Source: CAD feature listing. Evaluate the final solid. Frame: model axes, mm. Face numbers are marked on the shaded views. A direction names the side the tool comes from. Give positions to 0.01 mm unless a question says otherwise; leave off trailing zeros. Order: outer loops, then holes, each group sorted by start corner. A loop starts at its lowest first (then second) coordinate and runs counter-clockwise, first axis right, second up. Notation, with made-up numbers: M 86,-3.75 L 134,-3.75 A21 ccw 134,18.25 Z; hole C -17.5,38.5 d6. An arc over 180 degrees is marked long. Return JSON: item names as keys, results as strings.
from build123d import *

# Parameters (mm, degrees)
EXTRUDE_1_DEPTH             = 60
CUT_EXTRUDE_1_DEPTH         = 4
SKETCH_3_W                  = 5
SKETCH_3_H                  = 5
CUT_EXTRUDE_2_DEPTH         = 4
FILLET_1_R                  = 2
FILLET_2_R                  = 1
HOLE_WIZARD_M31_D           = 3.4
HOLE_WIZARD_M31_CBORE_D     = 6.5
HOLE_WIZARD_M31_CBORE_DEPTH = 3
SKETCH_9_W                  = 16.027024291
SKETCH_9_H                  = 8.780763308
CUT_EXTRUDE_4_DEPTH         = 6
SKETCH_10_R                 = 1.700955844
CUT_EXTRUDE_5_DEPTH         = 68.823299831


with BuildPart() as part:
    # Эскиз1 → Бобышка-Вытянуть1 (new body)
    with BuildSketch(Plane.XY):
        Polygon((-20, 5), (-15.381197846, -3), (-15.381197846, -4), (-30, -4), (-30, -6), (30, -6), (30, -4), (15.381197846, -4), (15.381197846, -3), (20, 5), (20, 6), (-20, 6), align=None)
    extrude(amount=EXTRUDE_1_DEPTH)

    # Эскиз2 → Вырез-Вытянуть1 (cut)
    with BuildSketch(Plane(origin=(0, 6, 0), x_dir=(1, 0, 0), z_dir=(0, 1, 0))):
        Polygon((15, 0), (-15, 0), (-15, -5), (-10.336923418, -15), (-10.336923418, -45), (-15, -55), (-15, -60), (15, -60), (15, -55), (10.336923418, -45), (10.336923418, -15), (15, -5), align=None)
    extrude(amount=-CUT_EXTRUDE_1_DEPTH, mode=Mode.SUBTRACT)

    # Эскиз3 → Вырез-Вытянуть2 (cut)
    with BuildSketch(Plane(origin=(0, 6, 0), x_dir=(1, 0, 0), z_dir=(0, 1, 0))):
        with Locations((-12.836923418, -30)):
            Rectangle(SKETCH_3_W, SKETCH_3_H)
        with Locations((12.836923418, -30)):
            Rectangle(SKETCH_3_W, SKETCH_3_H)
    extrude(amount=-CUT_EXTRUDE_2_DEPTH, mode=Mode.SUBTRACT)

    # Скругление1
    fillet_1_edges = [part.edges().sort_by_distance(p)[0] for p in [
        (20, 5.5, 0),
        (-20, 5.5, 0),
        (20, 5.5, 60),
        (-20, 5.5, 60),
        (-15, 4, 5),
        (-15, 4, 0),
        (15, 4, 0),
        (15, 4, 5),
        (10.336923418, 4, 15),
        (10.336923418, 4, 45),
        (15, 4, 55),
        (15, 4, 60),
        (-15, 4, 60),
        (-15, 4, 55),
    ]]
    fillet(fillet_1_edges, radius=FILLET_1_R)

    # Скругление2
    fillet_2_edges = [part.edges().sort_by_distance(p)[0] for p in [
        (-15.336923418, 4, 32.5),
        (-15.336923418, 4, 27.5),
        (10.336923418, 4, 27.5),
        (15.336923418, 4, 27.5),
        (15.336923418, 4, 32.5),
        (10.336923418, 4, 32.5),
    ]]
    fillet(fillet_2_edges, radius=FILLET_2_R)

    # Цековка для винта с внутренним шестигранником M31 (through all)
    with Locations(Plane(origin=(0, 2, 0), x_dir=(1, 0, 0), z_dir=(0, 1, 0))):
        with Locations((0, -24), (6, -30), (0, -36), (-6, -30)):
            CounterBoreHole(HOLE_WIZARD_M31_D / 2, HOLE_WIZARD_M31_CBORE_D / 2, HOLE_WIZARD_M31_CBORE_DEPTH)

    # Эскиз9 → Вырез-Вытянуть4 (cut)
    with BuildSketch(Plane(origin=(0, 2, 0), x_dir=(1, 0, 0), z_dir=(0, 1, 0))):
        with Locations((1.449252196, -53.358535403)):
            Rectangle(SKETCH_9_W, SKETCH_9_H)
    extrude(amount=-CUT_EXTRUDE_4_DEPTH, mode=Mode.SUBTRACT)

    # Эскиз10 → Вырез-Вытянуть5 (cut, through all)
    with BuildSketch(Plane(origin=(0, -4, 0), x_dir=(1, 0, 0), z_dir=(0, 1, 0))):
        with Locations(Location((-4.749733233, -52.305802454, 0), (0, 0, 180))):
            Circle(SKETCH_10_R)
    extrude(amount=-CUT_EXTRUDE_5_DEPTH, mode=Mode.SUBTRACT)


solid = part.part
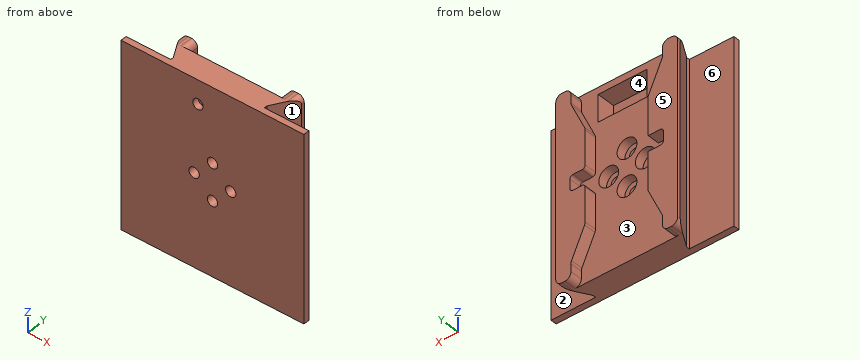
1. Draft query along X for the marked faces 1, 2, 3 and 4. Return one class per face: pulls with the +X half, pulls with the -X half, needs draft (parallel to the pull), parting line crosses it, or undercut.
Evaluation:
{"face 1": "pulls with the +X half", "face 2": "needs draft", "face 3": "undercut", "face 4": "undercut"}
2. Section query D-D (z = 13). Return loops of the section in (x, y).
Evaluation:
{"outline": "M -30,-6 L 30,-6 L 30,-4 L 15.38,-4 L 15.38,-3 L 20,5 L 20,6 L 11.27,6 L 11.27,2 L -11.27,2 L -11.27,6 L -20,6 L -20,5 L -15.38,-3 L -15.38,-4 L -30,-4 Z"}
3. Section query C-C (z = 37). Return loops of the section in (x, y), then the cut area to 3 significant figures.
Evaluation:
{"outline": "M -30,-6 L -1.37,-6 L -1.37,-1 L -3.09,-1 L -3.09,2 L -10.34,2 L -10.34,6 L -20,6 L -20,5 L -15.38,-3 L -15.38,-4 L -30,-4 Z; M 1.37,-6 L 30,-6 L 30,-4 L 15.38,-4 L 15.38,-3 L 20,5 L 20,6 L 10.34,6 L 10.34,2 L 3.09,2 L 3.09,-1 L 1.37,-1 Z", "area": "359 mm^2"}
4. Section query B-B (z = 30). State how many separate pieces and enclosed holes the cut face has, then the cut area to 3 significant figures.
Evaluation:
{"separate pieces": "3", "enclosed holes": "0", "area": "278 mm^2"}
5. Ray query, probe 1 along X at (y, z) = (-3.65, 30); probe 2 along Z at (x, y) = (-6, -0.2); probe 3 along Z at (x, y) = (6, -4.2). Return the intervals inside material, ascending.
Evaluation:
{"probe 1": "x = -15.38 to -7.7, -4.3 to 4.3, 7.7 to 15.38", "probe 2": "z = 0 to 26.75, 33.25 to 48.97, 57.75 to 60", "probe 3": "z = 0 to 28.3, 31.7 to 60"}
6. First-contact query: pin 1 (5 mm diameter, centred on y = 4.5, z = 46, fed in from -X); pin 2 (8.5 mm diameter, centred on x = -6, z = 30, fed in from +Y); pin 3 (5 mm diameter, centred on x = 6, z = 30, fed in from +Y). Flat tips, straight axial feed; report the tip coordinate or a pass-through.
Evaluation:
{"pin 1": "stops at x = -20", "pin 2": "stops at y = 2", "pin 3": "stops at y = -1"}
7. Section query A-A (x = 6). Return loops of the section in (y, z), then the cut area to 3 significant figures.
Evaluation:
{"outline": "M -6,0 L 2,0 L 2,26.75 L -1,26.75 L -1,28.3 L -6,28.3 Z; M -6,31.7 L -1,31.7 L -1,33.25 L 2,33.25 L 2,48.97 L -4,48.97 L -4,57.75 L 2,57.75 L 2,60 L -6,60 Z", "area": "391 mm^2"}
8. Set-up query: the marked faces 5 and 6. Return all of +Z, -Z, +X, -X, +Y, -Y with unobstructed straight access to the full face (end or side cutting, diameter ignored); none if empty.
Evaluation:
{"face 5": "+Z, -Z, +X, -X, +Y", "face 6": "+Z, -Z, -X"}
